Answer from the drawing. Dimensions are ordinates in mm from the lowest x, y and z of the part. Coordinates: 2 decimals unless noted, no trailing zeros. Write each loop counter-clockwise with the first axis right and the second up, starting at its lowest first coordinate (ties: lowest second). Pieces come first, ordered by that corner, then holes.
(1) For a pull along X with two mould halves and no side action, classify the marked faces 1, 2, 3 and 4 as +X half, -X half, draft (parallel to the pull), parting line (faces both ways), or undercut.
(2) Straight lines are drawn through the part: line 1 (X direction, y = 12.75, z = 41); line 2 (X direction, y = 20.5, z = 74.5); line 3 (Z direction, x = 65.5, y = 19.25). For each, find the intervals that lie inside material, in ascending order.
(3) The part is cut by section C-C on y = 8.5. Give the number of separate pieces and of enclosed holes in the cut face, plus the area to 3 significant figures.
(4) The part is cut by section B-B on x = 79. Determine the outline of the cut face in (y, z).
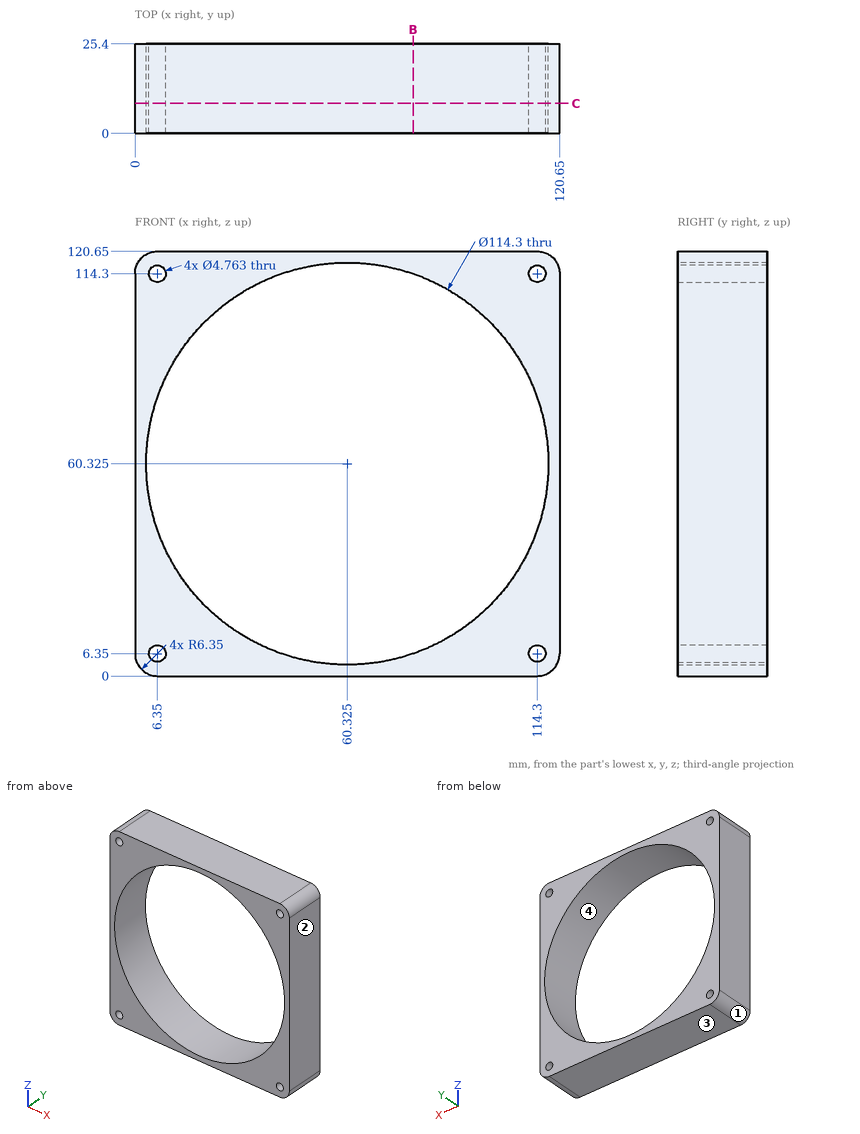
Model answer:
1. face 1: -X half
1. face 2: +X half
1. face 3: draft
1. face 4: undercut
2. line 1: x = 0 to 6.54, 114.11 to 120.65
2. line 2: x = 0 to 4.96, 115.69 to 120.65
2. line 3: z = 0 to 3.41, 117.24 to 120.65
3. separate pieces: 1
3. enclosed holes: 5
3. area: 4,190 mm2
4. outline: (0, 0) - (25.4, 0) - (25.4, 6.31) - (0, 6.31) - close; (0, 114.34) - (25.4, 114.34) - (25.4, 120.65) - (0, 120.65) - close
